from build123d import *

# Parameters (mm, degrees)
SKETCH1_W               = 50
SKETCH1_H               = 33
BOSS_EXTRUDE1_DEPTH     = 3
SKETCH2_W               = 50
SKETCH2_H               = 5
BOSS_EXTRUDE2_DEPTH     = 58.5
SKETCH6_W               = 50
SKETCH6_H               = 5
CUT_EXTRUDE3_DEPTH      = 3
SKETCH7_W               = 50
SKETCH7_H               = 11
BOSS_EXTRUDE4_DEPTH     = 15.5
CUT_EXTRUDE4_DEPTH      = 6
SKETCH4_R               = 2.2
CUT_EXTRUDE5_DEPTH      = 59.5
SKETCH3_R               = 2.2479
CUT_EXTRUDE1_DEPTH      = 24
CUT_EXTRUDE1_DEPTH_BACK = 6


with BuildPart() as part:
    # Sketch1 → Boss-Extrude1 (new body)
    with BuildSketch(Plane.XY):
        Rectangle(SKETCH1_W, SKETCH1_H)
    extrude(amount=BOSS_EXTRUDE1_DEPTH)

    # Sketch2 → Boss-Extrude2 (add)
    with BuildSketch(Plane.XY.offset(3)):
        with Locations((0, -14)):
            Rectangle(SKETCH2_W, SKETCH2_H)
    extrude(amount=BOSS_EXTRUDE2_DEPTH)

    # Sketch6 → Cut-Extrude3 (cut)
    with BuildSketch(Plane.XY.offset(3)):
        with Locations((0, 14)):
            Rectangle(SKETCH6_W, SKETCH6_H)
    extrude(amount=-CUT_EXTRUDE3_DEPTH, mode=Mode.SUBTRACT)

    # Sketch7 → Boss-Extrude4 (add)
    with BuildSketch(Plane(origin=(0, -11.5, 0), x_dir=(1, 0, 0), z_dir=(0, 1, 0))):
        with Locations((0, -8.5)):
            Rectangle(SKETCH7_W, SKETCH7_H)
    extrude(amount=BOSS_EXTRUDE4_DEPTH)

    # Sketch8 → Cut-Extrude4 (cut)
    with BuildSketch(Plane(origin=(0, 4, 0), x_dir=(1, 0, 0), z_dir=(0, 1, 0))):
        Polygon((-18, -3.4), (-22.416729559, -5.95), (-22.416729559, -11.05), (-18, -13.6), (-13.583270441, -11.05), (-13.583270441, -5.95), align=None)
        Polygon((13.583270441, -5.95), (18, -3.4), (22.416729559, -5.95), (22.416729559, -11.05), (18, -13.6), (13.583270441, -11.05), align=None)
    extrude(amount=-CUT_EXTRUDE4_DEPTH, mode=Mode.SUBTRACT)

    # Sketch4 → Cut-Extrude5 (cut, through all)
    with BuildSketch(Plane.XY.offset(3)):
        with Locations((-10.000570114, 0.5)):
            Circle(SKETCH4_R)
        with Locations((9.999429886, 0.5)):
            Circle(SKETCH4_R)
    extrude(amount=CUT_EXTRUDE5_DEPTH, mode=Mode.SUBTRACT)

    # Sketch3 → Cut-Extrude1 (cut, two sides)
    with BuildSketch(Plane(origin=(0, -11.5, 0), x_dir=(1, 0, 0), z_dir=(0, 1, 0))) as cut_extrude1_sk:
        with Locations((-18, -54.5)):
            Circle(SKETCH3_R)
        with Locations((18, -54.5)):
            Circle(SKETCH3_R)
        with Locations((-18, -8.5)):
            Circle(SKETCH3_R)
        with Locations((18, -8.5)):
            Circle(SKETCH3_R)
        with BuildLine():
            Line((-25, -51.5), (-25, -61.5))
            Line((-25, -61.5), (-15, -61.5))
            ThreePointArc((-15, -61.5), (-22.071067812, -58.571067812), (-25, -51.5))
        make_face()
        with BuildLine():
            Line((15, -61.5), (25, -61.5))
            Line((25, -61.5), (25, -51.5))
            ThreePointArc((25, -51.5), (22.071067812, -58.571067812), (15, -61.5))
        make_face()
    extrude(amount=CUT_EXTRUDE1_DEPTH, mode=Mode.SUBTRACT)
    extrude(cut_extrude1_sk.sketch, amount=-CUT_EXTRUDE1_DEPTH_BACK, mode=Mode.SUBTRACT)


solid = part.part
Build history of the part. All positions in model axes, mm. A direction names the side the tool comes from. Coordinates: 2 decimals unless noted, no trailing zeros. Order: outer loops, then holes, each group sorted by start corner. A loop starts at its lowest first (then second) coordinate and runs counter-clockwise, first axis right, second up. Notation, with made-up numbers: (1, 19) - (18, 19) arc R22 ccw to (18, 55) - close; hole circle Ø3 at (19, 43). An arc over 180 degrees is marked (long way). Write each question's results on one line, items separated by ' | '. Start each with the question number.
Item 1: Band-saw the part on A-A on z = 8.5. Write the cut outline in (x, y).
Item 2: Band-saw the part on B-B on x = 7. Write the cut outline in (y, z).
Item 3: Mould opens along X. For faces 1 (the face through (22.15, -13.96, 58.49)), 2 (the face through (7.8, 0.6, 8.4)), 3 (the face through (0, 8, 3)) say: released by +X, released by -X, zero draft, split by the parting line, or undercut.
Item 4: Band-saw the part on D-D on y = -14. Write the cut outline in (x, z), and give its area (3 significant figures).
Item 5: Tool access for faces 4 (the face through (13.583, 1, 9)), 5 (the face through (19.2, -9.1, 6.6)), 6 (the face through (0, -11.5, 37)): list every direction of +Z, -Z, +X, -X, +Y, -Y with a clear straight run to the whole face (end or side of a thin tool).
Item 6: Band-saw the part on C-C on y = -9.75. Write the cut outline in (x, z).
Item 7: Flat gauge pins, fed straight in: pin 1 (5 mm diameter, centred on x = 10, y = 0.5, fed in from +Z); pin 2 (5 mm diameter, centred on x = -9, z = 35, fed in from +Y); pin 3 (5 mm diameter, centred on x = 18, z = 8.5, fed in from +Y). Where does each tip first touch, or does it go through?
Item 8: Wall check: probe 1 along X at (y, z) = (0.5, 6.25); probe 2 along Z at (x, y) = (-18, -5.25); probe 3 along X at (y, z) = (-7, 9.5). Give the ranges that are in metal, low to high. Write a range as [from, to].
Numbers:
1) outline: (-25, -16.5) - (-20.25, -16.5) - (-20.25, -2) - (-22.42, -2) - (-22.42, 4) - (-25, 4) - close; (-15.75, -16.5) - (15.75, -16.5) - (15.75, -2) - (13.58, -2) - (13.58, 4) - (-13.58, 4) - (-13.58, -2) - (-15.75, -2) - close; (20.25, -16.5) - (25, -16.5) - (25, 4) - (22.42, 4) - (22.42, -2) - (20.25, -2) - close; hole circle Ø4.4 at (-10, 0.5); hole circle Ø4.4 at (10, 0.5)
2) outline: (-16.5, 0) - (11.5, 0) - (11.5, 3) - (4, 3) - (4, 14) - (-11.5, 14) - (-11.5, 61.5) - (-16.5, 61.5) - close
3) face 1: released by +X | face 2: undercut | face 3: zero draft
4) outline: (-25, 0) - (25, 0) - (25, 51.5) arc R10 ccw to (15, 61.5) - (-15, 61.5) arc R10 ccw to (-25, 51.5) - close; hole circle Ø4.5 at (-18, 8.5); hole circle Ø4.5 at (-18, 54.5); hole circle Ø4.5 at (18, 8.5); hole circle Ø4.5 at (18, 54.5) | area: 2,970 mm^2
5) face 4: +Y | face 5: +Y, -Y | face 6: +Z, +X, -X, +Y
6) outline: (-25, 0) - (25, 0) - (25, 14) - (-25, 14) - close; hole circle Ø4.5 at (-18, 8.5); hole circle Ø4.5 at (18, 8.5)
7) pin 1: z = 14 | pin 2: y = -11.5 | pin 3: y = -2
8) probe 1: [-25, -22.42], [-13.58, -12.2], [-7.8, 7.8], [12.2, 13.58], [22.42, 25] | probe 2: [0, 6.25], [10.75, 14] | probe 3: [-25, -20.01], [-15.99, 15.99], [20.01, 25]
